from build123d import *

# Parameters (mm, degrees)
SKETCH1_R           = 5
SKETCH1_R_2         = 4
BOSS_EXTRUDE1_DEPTH = 2
BOSS_EXTRUDE2_START = -1.9
SKETCH2_R           = 4
SKETCH2_R_2         = 3
BOSS_EXTRUDE2_DEPTH = 1.9
BOSS_EXTRUDE4_START = 0.1
SKETCH3_R           = 4
BOSS_EXTRUDE4_DEPTH = 0.1
SKETCH4_R           = 4
CUT_EXTRUDE1_DEPTH  = 1


with BuildPart() as part:
    # Sketch1 → Boss-Extrude1 (new body)
    with BuildSketch(Plane(origin=(0, 0, 0), x_dir=(1, 0, 0), z_dir=(0, 1, 0))):
        with Locations(Location((0, 0, 0), (0, 0, 270))):
            Circle(SKETCH1_R)
        with Locations(Location((0, 0, 0), (0, 0, 270))):
            Circle(SKETCH1_R_2, mode=Mode.SUBTRACT)
    extrude(amount=BOSS_EXTRUDE1_DEPTH)

    # Sketch2 → Boss-Extrude2 (add)
    with BuildSketch(Plane(origin=(0, 2, 0), x_dir=(1, 0, 0), z_dir=(0, 1, 0)).offset(BOSS_EXTRUDE2_START)):
        with Locations(Location((0, 0, 0), (0, 0, 270))):
            Circle(SKETCH2_R)
        with Locations(Location((0, 0, 0), (0, 0, 270))):
            Circle(SKETCH2_R_2, mode=Mode.SUBTRACT)
    extrude(amount=BOSS_EXTRUDE2_DEPTH)

    # Sketch3 → Boss-Extrude4 (add)
    with BuildSketch(Plane.XZ.offset(-0.1).offset(BOSS_EXTRUDE4_START)):
        Circle(SKETCH3_R)
    extrude(amount=-BOSS_EXTRUDE4_DEPTH)

    # Sketch4 → Cut-Extrude1 (cut)
    with BuildSketch(Plane.XZ):
        with Locations(Location((0, 0, 0), (0, 0, 270))):
            Circle(SKETCH4_R)
    extrude(amount=-CUT_EXTRUDE1_DEPTH, mode=Mode.SUBTRACT)


solid = part.part
Part model, mm, in its own coordinate system. Coordinates: 2 decimals unless noted, no trailing zeros. Loops run counter-clockwise (first coordinate to the right, second up) from the corner with the lowest first, then second, coordinate; pieces in that order, holes last. Notation, with made-up numbers: M 2.5,58 L 30.5,58 A17 cw 30.5,78 Z; hole C -27.5,-18.75 d7. An arc over 180 degrees is marked long. Use a Markdown table: item, result. Add a question column.
Q1. Cut at A-A (z = 0). Write the cut outline in (x, y), and give its area (3 significant figures).
Q2. Cut at D-D (x = -3.5). Write the cut outline in (y, z).
Q3. Cut at C-C (y = 1.3). Write the cut outline in (x, z), and give its area (3 significant figures).
Q4. Pin check, flat tips, straight feed: P1, Ø5, axis at x = 1.5, z = 2.5, coming from the -Y side; P2, Ø2.5, axis at x = 1, z = -1, coming from the -Y side. Stop position of each tip, or through.
Q5. Cut at B-B (x = 0). Write the cut outline in (y, z).
Q6. Probe L1, parallel to X at y = 0.65, z = 0; L2, parallel to X at y = 1.45, z = 0; L3, parallel to Z at x = -2, y = 1.35. List the from-to ranges inside material, lowest first.
Q7. Mould opens along X. For faces 1 (the cylindrical face through (-4.88, 0.99, -1.08)), 2 (the cylindrical face through (-3.905, 0.493, 0.867)), 3 (the flat face through (-3.3, 2, -0.1)), 4 (the cylindrical face through (0.9, 1.49, 2.86)) say: +X half, -X half, draft (parallel to the pull), parting line (faces both ways), or undercut.
Worked out:
| question | item | result |
|---|---|---|
| 1 | outline | M -5,0 L -4,0 L -4,1 L -3,1 L -3,2 L -5,2 Z; M 3,1 L 4,1 L 4,0 L 5,0 L 5,2 L 3,2 Z |
| 1 | area | 6.00 mm2 |
| 2 | outline | M 0,-3.57 L 2,-3.57 L 2,3.57 L 0,3.57 L 0,1.94 L 1,1.94 L 1,-1.94 L 0,-1.94 Z |
| 3 | outline | C 0,0 d10; hole C 0,0 d6 |
| 3 | area | 50.3 mm2 |
| 4 | P1 | stops at y = 0 |
| 4 | P2 | passes through |
| 5 | outline | M 0,-5 L 2,-5 L 2,-3 L 1,-3 L 1,-4 L 0,-4 Z; M 0,4 L 1,4 L 1,3 L 2,3 L 2,5 L 0,5 Z |
| 6 | L1 | x = -5 to -4, 4 to 5 |
| 6 | L2 | x = -5 to -3, 3 to 5 |
| 6 | L3 | z = -4.58 to -2.24, 2.24 to 4.58 |
| 7 | face 1 | parting line |
| 7 | face 2 | undercut |
| 7 | face 3 | draft |
| 7 | face 4 | undercut |
